```python
from build123d import *

# Parameters (mm, degrees)
SKETCH_1_W          = 60
SKETCH_1_H          = 20
SKETCH_1_R          = 1.5
SKETCH_1_R_2        = 1.8
EXTRUDE_1_DEPTH     = 3
SKETCH_7_W          = 60
SKETCH_7_H          = 10
EXTRUDE_3_DEPTH     = 19
SKETCH_8_R          = 1.8
CUT_EXTRUDE_3_DEPTH = 46.692815914
SKETCH_9_W          = 6
SKETCH_9_H          = 19
EXTRUDE_4_DEPTH     = 2
SKETCH_10_W         = 40
SKETCH_10_H         = 7
CUT_EXTRUDE_4_DEPTH = 48.019500488
FILLET_2_R          = 2


with BuildPart() as part:
    # ｽｹｯﾁ1 → ﾎﾞｽ - 押し出し1 (new body)
    with BuildSketch(Plane(origin=(0, 0, 0), x_dir=(1, 0, 0), z_dir=(0, 1, 0))):
        with Locations((2.380597015, -16.044776119)):
            Rectangle(SKETCH_1_W, SKETCH_1_H)
        with Locations(Location((-22.119402985, -21.044776119, 0), (0, 0, 270))):
            Circle(SKETCH_1_R, mode=Mode.SUBTRACT)
        with Locations(Location((26.880597015, -21.044776119, 0), (0, 0, 270))):
            Circle(SKETCH_1_R, mode=Mode.SUBTRACT)
        with Locations(Location((-22.619402985, -11.044776119, 0), (0, 0, 270))):
            Circle(SKETCH_1_R_2, mode=Mode.SUBTRACT)
        with Locations(Location((27.380597015, -11.044776119, 0), (0, 0, 270))):
            Circle(SKETCH_1_R_2, mode=Mode.SUBTRACT)
    extrude(amount=EXTRUDE_1_DEPTH)

    # ｽｹｯﾁ7 → ﾎﾞｽ - 押し出し3 (add)
    with BuildSketch(Plane(origin=(0, 3, 0), x_dir=(1, 0, 0), z_dir=(0, 1, 0))):
        with Locations((2.380597015, -11.044776119)):
            Rectangle(SKETCH_7_W, SKETCH_7_H)
    extrude(amount=EXTRUDE_3_DEPTH)

    # ｽｹｯﾁ8 → ｶｯﾄ - 押し出し3 (cut, through all)
    with BuildSketch(Plane.XZ.offset(-3)):
        with Locations(Location((27.380597015, 11.044776119, 0), (0, 0, 270))):
            Circle(SKETCH_8_R)
        with Locations(Location((-22.619402985, 11.044776119, 0), (0, 0, 270))):
            Circle(SKETCH_8_R)
    extrude(amount=-CUT_EXTRUDE_3_DEPTH, mode=Mode.SUBTRACT)

    # ｽｹｯﾁ9 → ﾎﾞｽ - 押し出し4 (add)
    with BuildSketch(Plane.XY.offset(16.044776119)):
        with Locations((29.380597015, 12.5)):
            Rectangle(SKETCH_9_W, SKETCH_9_H)
        with Locations((-24.619402985, 12.5)):
            Rectangle(SKETCH_9_W, SKETCH_9_H)
    extrude(amount=EXTRUDE_4_DEPTH)

    # ｽｹｯﾁ10 → ｶｯﾄ - 押し出し4 (cut, through all)
    with BuildSketch(Plane(origin=(0, 22, 0), x_dir=(1, 0, 0), z_dir=(0, 1, 0))):
        with Locations((2.380597015, -9.544776119)):
            Rectangle(SKETCH_10_W, SKETCH_10_H)
    extrude(amount=-CUT_EXTRUDE_4_DEPTH, mode=Mode.SUBTRACT)

    # ﾌｨﾚｯﾄ2
    fillet_2_edges = [part.edges().sort_by_distance(p)[0] for p in [
        (32.380597015, 12.5, 18.044776119),
        (26.380597015, 12.5, 18.044776119),
        (-27.619402985, 12.5, 18.044776119),
        (-21.619402985, 12.5, 18.044776119),
        (32.380597015, 1.5, 26.044776119),
        (-27.619402985, 1.5, 26.044776119),
        (-27.619402985, 11, 6.044776119),
        (32.380597015, 11, 6.044776119),
        (22.380597015, 11, 6.044776119),
        (22.380597015, 11, 13.044776119),
        (-17.619402985, 11, 13.044776119),
        (-17.619402985, 11, 6.044776119),
    ]]
    fillet(fillet_2_edges, radius=FILLET_2_R - 0.0001)  # a hair under: the kernel refuses the full size


solid = part.part
```
For this review, take the finished solid that the model builds, in its own axes (mm). A direction names the side the tool comes from. Coordinates: 2 decimals unless noted, no trailing zeros. Write each loop counter-clockwise with the first axis right and the second up, starting at its lowest first coordinate (ties: lowest second). Pieces come first, ordered by that corner, then holes. Notation, with made-up numbers: (62.25, -11.5) -> (103.25, -11.5) arc R16 ccw to (103.25, -1.5) -> close; hole circle Ø4 at (-0.75, 40.25). An arc over 180 degrees is marked (long way). Put each result on its own line as item: value.
Q1. Clearance check with flat-ended pins moving along their axes: pin 1 Ø5 at (x, z) = (26.88, 21.04) entering from +Y; pin 2 Ø2 at (x, y) = (-25, 9.5) entering from +Z; pin 3 Ø3.5 at (x, z) = (-22.12, 21.04) entering from -Y; pin 4 Ø3 at (x, z) = (-22.62, 11.04) entering from +Y. State where each tip first meets the part, or that it passes through.
From the geometry:
pin 1: stops at y = 3
pin 2: stops at z = 18.04
pin 3: stops at y = 0
pin 4: passes through
Q2. Take a section at B-B, the plane y = 9.5. Count the separate pieces of the cut face and the enclosed holes in it, then the cut area to 3 significant figures.
From the geometry:
separate pieces: 1
enclosed holes: 2
area: 318 mm2
Q3. Tool access review of faces 1 (the flat face through (2, 12, 16.045)), 2 (the cylindrical face through (-27.05, 1.52, 25.44)), 3 (the cylindrical face through (31.779, 12.633, 17.474)), 4 (the cylindrical face through (23, 10.8, 6.6)), 5 (the cylindrical face through (-27, 10.8, 6.6)): name each direction out of +Z, -Z, +X, -X, +Y, -Y from which nothing blocks a thin tool from reaching the whole face with its end or side.
From the geometry:
face 1: +Z, +Y
face 2: +Z, -X, +Y, -Y
face 3: +Z, +X, +Y
face 4: -Z, +Y, -Y
face 5: -Z, -X, +Y, -Y
Q4. Take a section at A-A, the plane z = 12.25. State the section outline as (x, y) points, then the cut area to 3 significant figures.
From the geometry:
outline: (-27.62, 0) -> (-23.96, 0) -> (-23.96, 22) -> (-27.62, 22) -> close; (-21.28, 0) -> (-17.22, 0) -> (-17.22, 22) -> (-21.28, 22) -> close; (21.98, 0) -> (26.04, 0) -> (26.04, 22) -> (21.98, 22) -> close; (28.72, 0) -> (32.38, 0) -> (32.38, 22) -> (28.72, 22) -> close
area: 340 mm2
Q5. Take a section at C-C, the plane y = 2. State the section outline as (x, z) points.
From the geometry:
outline: (-27.62, 8.04) arc R2 ccw to (-25.62, 6.04) -> (-19.62, 6.04) arc R2 ccw to (-17.62, 8.04) -> (-17.62, 11.04) arc R2 cw to (-15.62, 13.04) -> (20.38, 13.04) arc R2 cw to (22.38, 11.04) -> (22.38, 8.04) arc R2 ccw to (24.38, 6.04) -> (30.38, 6.04) arc R2 ccw to (32.38, 8.04) -> (32.38, 24.04) arc R2 ccw to (30.38, 26.04) -> (-25.62, 26.04) arc R2 ccw to (-27.62, 24.04) -> close; hole circle Ø3.6 at (-22.62, 11.04); hole circle Ø3 at (-22.12, 21.04); hole circle Ø3 at (26.88, 21.04); hole circle Ø3.6 at (27.38, 11.04)
Q6. Wall thickness on L1, parallel to X at y = 13.25, z = 11; L2, parallel to Z at x = -12, y = 5; L3, parallel to Y at x = 22.5, z = 17.75: over which ranges is each line inside the solid? List them lowest first.
From the geometry:
L1: x = -27.62 to -24.42, -20.82 to -17.62, 22.38 to 25.58, 29.18 to 32.38
L2: z = 13.04 to 16.04
L3: y = 0 to 3
Q7. Take a section at D-D, the plane x = 5. State the section outline as (y, z) points, then the cut area to 3 significant figures.
From the geometry:
outline: (0, 13.04) -> (22, 13.04) -> (22, 16.04) -> (3, 16.04) -> (3, 26.04) -> (0, 26.04) -> close
area: 96.0 mm2
Q8. The part is to be moulded in two halves that separate along Z. For faces 6 (the cylindrical face through (28.145, 1.479, 21.851)), 7 (the cylindrical face through (-27.05, 12.63, 17.44)), 8 (the cylindrical face through (31.81, 10.846, 6.646)), 9 (the flat face through (-27.619, 11, 13)), say which applies: +Z half, -Z half, draft (parallel to the pull), parting line (faces both ways), or undercut.
From the geometry:
face 6: undercut
face 7: +Z half
face 8: -Z half
face 9: draft
